Verification items for the finished model (mm, model axes). Face numbers are marked on the shaded views. A direction names the side the tool comes from. Give positions to 0.01 mm unless a question says otherwise; leave off trailing zeros. Write each loop counter-clockwise with the first axis right and the second up, starting at its lowest first coordinate (ties: lowest second). Pieces come first, ordered by that corner, then holes. Notation, with made-up numbers: (75.25, 2.5) - (82.25, 2.5) arc R22 cw to (82.25, 30.5) - close; hole circle Ø3 at (23, -26). An arc over 180 degrees is marked (long way). Answer as a JSON object with one key per item and string values. Group by question number.
Item 1: Go/stop test with flat-tipped pins: pin 1 (3 mm diameter, centred on x = 4.5, y = 8.5, fed in from -Z); pin 2 (6 mm diameter, centred on y = -3, z = 8, fed in from +X); pin 3 (3 mm diameter, centred on y = 9, z = 2.5, fed in from +X). Record where each tip stops, or that it passes through.
Item 2: Draft check along X on the marked faces 4, 5 and 6. Enter one of: +X half, -X half, draft (parallel to the pull), parting line (faces both ways), or undercut.
Item 3: Tool access check on the marked faces 1, 2 and 3. Record the directions out of +Z, -Z, +X, -X, +Y, -Y that give a thin tool (end or side, any length) a straight path to the whole face; none if there is none.
Item 4: Sectioned sample at B-B, the plane x = -23. Record the boundary of the cut face in (y, z), and give its area (3 significant figures).
Item 5: Scan lines: line 1 along X through (y, z) = (0, 3.2); line 2 along X through (y, z) = (0, 6.55); line 3 along Y through (x, z) = (23, 7.5). Record each from-to range of solid material in increasing order. Write a range as [from, to].
Item 6: Sectioned sample at D-D, the plane x = 10.5. Record the boundary of the cut face in (y, z), and give its area (4 significant figures).
Item 7: Sectioned sample at C-C, the plane y = 0. Record the boundary of the cut face in (x, z), and give its area (3 significant figures).
Item 8: Sectioned sample at A-A, the plane z = 3. Record the boundary of the cut face in (x, y).
Autodesk Inventor part; units mm, degrees
ref_plane "YZ Plane" through (0, 0, 0) normal (1, 0, 0) x (0, 1, 0)
ref_plane "XZ Plane" through (0, 0, 0) normal (0, 1, 0) x (-1, 0, 0)
ref_plane "XY Plane" through (0, 0, 0) normal (0, 0, 1) x (1, 0, 0)
sketch "Náčrt1" plane through (0, 0, 0) normal (0, 0, 1) x (1, 0, 0)
  line L0 (-24.5, 0) -> (24.5, 0)
  line L1 (0, -14) -> (0, 14)
  line L2 (-17.5, 10) -> (17.5, 10)
  line L3 (17.5, 10) -> (17.5, -10)
  line L4 (17.5, -10) -> (-17.5, -10)
  line L5 (-17.5, -10) -> (-17.5, 10)
  point P0 (0, 0)
  point P1 (0, 10)
  point P2 (17.5, 0)
  point P3 (-17.5, 0)
  point P4 (0, -10)
  dimension "d0" = 35
  dimension "d1" = 20
extrude "Vysunutí1" add sketch "Náčrt1" along normal blind 10
sketch "Náčrt2" plane through (0, 0, 0) normal (0, 0, -1) x (-1, 0, 0)
  line L0 (17.5, -10) -> (-17.5, -10)
  line L1 (17.5, 10) -> (17.5, -10)
  line L2 (-17.5, 10) -> (17.5, 10)
  line L3 (-17.5, -10) -> (-17.5, 10)
  line L4 (-15, 7.5) -> (15, 7.5)
  line L5 (15, 7.5) -> (15, -7.5)
  line L6 (15, -7.5) -> (-15, -7.5)
  line L7 (-15, -7.5) -> (-15, 7.5)
  line L8 (24.5, 0) -> (-24.5, 0)
  line L9 (0, -14) -> (0, 14)
  point P0 (0, 0)
  point P1 (0, 7.5)
  point P2 (15, 0)
  dimension "d4" = 15
  dimension "d5" = 30
extrude "Vysunutí2" cut sketch "Náčrt2" against normal blind 7.5 contours L9 L8 L5 L6 | L6 L7 L8 L9 | L8 L9 L4 L5 | L8 L7 L4 L9
sketch "Náčrt3" plane through (-17.5, 10, 0) normal (0, 1, 0) x (1, 0, 0)
  line L0 (35, 0) -> (0, 0)
  line L1 (0, 0) -> (0, -10)
  line L2 (35, -10) -> (0, -10)
  line L3 (35, 0) -> (35, -10)
  line L4 (30, -5) -> (5, -5)
  line L5 (5, -5) -> (5, 0)
  line L6 (5, 0) -> (30, 0)
  line L7 (30, 0) -> (30, -5)
  point P0 (17.5, 0)
  point P1 (17.5, 0)
  point P2 (30, 0)
  point P3 (5, 0)
  dimension "d8" = 5
  dimension "d9" = 25
extrude "Vysunutí3" cut sketch "Náčrt3" against normal through all contours L7 L4 L5 L0
sketch "Náčrt4" plane through (0, 0, 0) normal (0, 0, -1) x (-1, 0, 0)
  line L0 (-12.5, 7.5) -> (-12.5, 10)
  line L1 (-17.5, 10) -> (-12.5, 10)
  line L2 (-17.5, -10) -> (-17.5, 10)
  line L3 (-12.5, -10) -> (-17.5, -10)
  line L4 (-12.5, -10) -> (-12.5, -7.5)
  line L5 (-12.5, -7.5) -> (-15, -7.5)
  line L6 (-15, -7.5) -> (-15, 7.5)
  line L7 (-15, 7.5) -> (-12.5, 7.5)
  line L8 (12.5, 10) -> (12.5, 7.5)
  line L9 (12.5, 7.5) -> (15, 7.5)
  line L10 (15, 7.5) -> (15, -7.5)
  line L11 (15, -7.5) -> (12.5, -7.5)
  line L12 (12.5, -7.5) -> (12.5, -10)
  line L13 (17.5, -10) -> (12.5, -10)
  line L14 (17.5, 10) -> (17.5, -10)
  line L15 (12.5, 10) -> (17.5, 10)
  line L16 (52.5, 0) -> (-52.5, 0)
  line L17 (0, -14) -> (0, 14)
  line L18 (-17.5, 10) -> (17.5, 10)
  line L19 (-27.5, 10) -> (-17.5, 10)
  line L20 (-17.5, 10) -> (-17.5, -10)
  line L21 (-17.5, -10) -> (-27.5, -10)
  line L22 (-27.5, -10) -> (-27.5, 10)
  line L23 (17.5, 10) -> (27.5, 10)
  line L24 (27.5, 10) -> (27.5, -10)
  line L25 (27.5, -10) -> (17.5, -10)
  line L26 (17.5, -10) -> (17.5, 10)
  arc A0 (-27.5, 10) -> (-27.5, -10) centre (-10, 0) ccw
  arc A1 (27.5, -10) -> (27.5, 10) centre (10, 0) ccw
  point P0 (0, 0)
  point P1 (-17.5, 0)
  point P2 (17.5, 0)
  point P3 (-17.5, 0)
  point P4 (17.5, 0)
  dimension "d26" = 10
  dimension "d27" = 10
  dimension "d32" = 10
  dimension "d33" = 10
extrude "Vysunutí4" add sketch "Náčrt4" against normal up to surface (10 mm away) contours L2 L16 L22 L19 | L2 L21 L22 L16 | L22 L16 A0 | L22 A0 L16 | L23 L24 L16 L14 | L16 L24 L25 L14 | A1 L16 L24 | L16 A1 L24
sketch "Náčrt5" plane through (0, 0, 10) normal (0, 0, 1) x (1, 0, 0)
  line L0 (-47.1525, 0) -> (47.1525, 0)
  line L1 (0, -14) -> (0, 14)
  line L2 (-27.5, 10) -> (27.5, 10)
  line L3 (27.5, -10) -> (-27.5, -10)
  arc A0 (27.5, -10) -> (27.5, 10) centre (10, 0) ccw
  arc A1 (-27.5, 10) -> (-27.5, -10) centre (-10, 0) ccw
  point P0 (0, 0)
  point P1 (23, 0)
  point P2 (-23, 0)
  dimension "d30" = 46
  dimension "d31" = 23
hole "Díra1" at (23, 0, 10) at (-23, 0, 10) direction (0, 0, -1) diameter 4.5 end through all counterbore diameter 8 counterbore depth 4.6
fillet "Zaoblení2" radius 5 4 edges at (27.5, 10, 5) (-27.5, 10, 5) (-27.5, -10, 5) (27.5, -10, 5)
chamfer "Zkosení1" distance 0.5 angle 45 2 edges at (0, 10, 10) (0, -10, 10)
properties part number "drzak_kable_horni_dil"
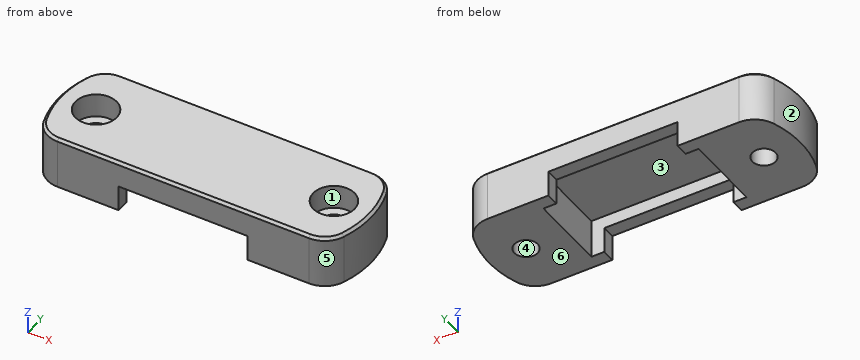
Geometry check:
{
 "1": {"pin 1": "z = 5", "pin 2": "x = 30.16", "pin 3": "x = 28.64"},
 "2": {"face 4": "undercut", "face 5": "+X half", "face 6": "draft"},
 "3": {"face 1": "+Z", "face 2": "+Z, -Z, -X", "face 3": "-Z"},
 "4": {"outline": "(-10, 0) - (-2.25, 0) - (-2.25, 5.4) - (-4, 5.4) - (-4, 10) - (-9.5, 10) - (-10, 9.5) - close; (2.25, 0) - (10, 0) - (10, 9.5) - (9.5, 10) - (4, 10) - (4, 5.4) - (2.25, 5.4) - close", "area": "139 mm^2"},
 "5": {"line 1": "[-30.16, -25.25], [-20.75, -15], [15, 20.75], [25.25, 30.16]", "line 2": "[-30.16, -27], [-19, -15], [15, 19], [27, 30.16]", "line 3": "[-10, -4], [4, 10]"},
 "6": {"outline": "(-10, 5) - (-7.5, 5) - (-7.5, 7.5) - (7.5, 7.5) - (7.5, 5) - (10, 5) - (10, 9.5) - (9.5, 10) - (-9.5, 10) - (-10, 9.5) - close", "area": "62.25 mm^2"},
 "7": {"outline": "(-30.16, 0) - (-25.25, 0) - (-25.25, 5.4) - (-27, 5.4) - (-27, 10) - (-29.66, 10) - (-30.16, 9.5) - close; (-20.75, 0) - (-15, 0) - (-15, 7.5) - (15, 7.5) - (15, 0) - (20.75, 0) - (20.75, 5.4) - (19, 5.4) - (19, 10) - (-19, 10) - (-19, 5.4) - (-20.75, 5.4) - close; (25.25, 0) - (30.16, 0) - (30.16, 9.5) - (29.66, 10) - (27, 10) - (27, 5.4) - (25.25, 5.4) - close", "area": "256 mm^2"},
 "8": {"outline": "(-29.03, -6.65) arc R5 ccw to (-24.31, -10) - (-12.5, -10) - (-12.5, -7.5) - (-15, -7.5) - (-15, 7.5) - (-12.5, 7.5) - (-12.5, 10) - (-24.31, 10) arc R5 ccw to (-29.03, 6.65) arc R20.16 ccw to start; (12.5, -10) - (24.31, -10) arc R5 ccw to (29.03, -6.65) arc R20.16 ccw to (29.03, 6.65) arc R5 ccw to (24.31, 10) - (12.5, 10) - (12.5, 7.5) - (15, 7.5) - (15, -7.5) - (12.5, -7.5) - close; hole circle Ø4.5 at (-23, 0); hole circle Ø4.5 at (23, 0)"}
}
